```python
from build123d import *

# Parameters (mm, degrees)
EXTRUDE_1_DEPTH     = 6.5
SKETCH_2_R          = 8.75
EXTRUDE_2_DEPTH     = 3
SKETCH_3_R          = 10
EXTRUDE_3_DEPTH     = 12.5
CHAMFER_1_SIZE      = 1.5
SKETCH_6_R          = 5
CUT_EXTRUDE_1_DEPTH = 29.172880507
CHAMFER_2_SIZE      = 0.5


with BuildPart() as part:
    # 草图1 → 凸台-拉伸1 (new body)
    with BuildSketch(Plane(origin=(0, 0, 0), x_dir=(1, 0, 0), z_dir=(0, 1, 0))):
        Polygon((6.553289027, 11.549360859), (-6.725395388, 11.449995205), (-13.278684415, -0.099365654), (-6.553289027, -11.549360859), (6.725395388, -11.449995205), (13.278684415, 0.099365654), align=None)
    extrude(amount=EXTRUDE_1_DEPTH)

    # 草图2 → 凸台-拉伸2 (add)
    with BuildSketch(Plane(origin=(0, 6.5, 0), x_dir=(1, 0, 0), z_dir=(0, 1, 0))):
        with Locations(Location((0, 0, 0), (0, 0, 270))):
            Circle(SKETCH_2_R)
    extrude(amount=EXTRUDE_2_DEPTH)

    # 草图3 → 凸台-拉伸3 (add)
    with BuildSketch(Plane(origin=(0, 9.5, 0), x_dir=(1, 0, 0), z_dir=(0, 1, 0))):
        with Locations(Location((0, 0, 0), (0, 0, 270))):
            Circle(SKETCH_3_R)
    extrude(amount=EXTRUDE_3_DEPTH)

    # 倒角1
    chamfer_1_edges = [part.edges().sort_by_distance(p)[0] for p in [
        (0, 22, -10),
    ]]
    chamfer(chamfer_1_edges, length=CHAMFER_1_SIZE)

    # 草图5 → 切除-旋转3 (revolve, cut)
    with BuildSketch(Plane(origin=(0, 0, 0), x_dir=(0.49350563267132574, 0, -0.8697426001534446), z_dir=(0.8697426001534445, 0, 0.4935056326713257)), mode=Mode.PRIVATE) as cut_revolve_3_sk:
        Polygon((13.279056191, 1), (11.279056191, 0), (13.279056191, 0), align=None)
    revolve(cut_revolve_3_sk.sketch.rotate(Axis((0, -1000, 0), (0, 1, 0)), 180.000000003), axis=Axis((0, -1000, 0), (0, 1, 0)), mode=Mode.SUBTRACT)

    # 草图6 → 切除-拉伸1 (cut, through all)
    with BuildSketch(Plane(origin=(0, 22, 0), x_dir=(1, 0, 0), z_dir=(0, 1, 0))):
        with Locations(Location((0, 0, 0), (0, 0, 270))):
            Circle(SKETCH_6_R)
    extrude(amount=-CUT_EXTRUDE_1_DEPTH, mode=Mode.SUBTRACT)

    # 倒角2
    chamfer_2_edges = [part.edges().sort_by_distance(p)[0] for p in [
        (0, 0, -5),
        (0, 22, -5),
    ]]
    chamfer(chamfer_2_edges, length=CHAMFER_2_SIZE)


solid = part.part
```
Verification items for the finished model (mm, model axes). A direction names the side the tool comes from. Round coordinates to 2 decimals unless told otherwise and drop trailing zeros. Write each loop counter-clockwise with the first axis right and the second up, starting at its lowest first coordinate (ties: lowest second). Pieces come first, ordered by that corner, then holes.
1. Access from +Z, -Z, +X, -X, +Y, -Y to the whole of each face (thin tool, end or side, straight path). Record for faces 1 (the cylindrical face through (-9.76, 14.92, -2.17)), 2 (the cylindrical face through (-5.324, 7.979, -6.944)), 3 (the flat face through (-6, 22, 0)).
2. Section check B-B on x = 0. Enter the section's corners in (y, z).
3. Section check C-C on y = 10.5. Enter the section's corners in (x, z), plus the area to 3 significant figures.
4. Scan lines: L1, parallel to X at y = 14, z = 0; L2, parallel to X at y = 9.25, z = 0; L3, parallel to Y at x = -8.5, z = -4.5. Record each from-to range of solid material in increasing order.
5. Draft check along Z on faces 4 (the flat face through (-9.963, 3.261, 5.744)), 5 (the flat face through (-9, 9.5, 0)), 6 (the cylindrical face through (-4.88, 11.15, -1.08)). Enter one of: +Z half, -Z half, draft (parallel to the pull), parting line (faces both ways), or undercut.
6. Section check A-A on y = 5.5. Enter the section's corners in (x, z).
7. Gauge pin test, flat ends, axial feed: P1, Ø1.5, axis at y = 6, z = -6, coming from the +X side; P2, Ø10, axis at y = 6, z = -7, coming from the +X side; P3, Ø6, axis at x = 7, y = 15, coming from the +Z side. Record the tip position at first contact, or that the pin passes through.
Answer:
1. face 1: +Y
1. face 2: none
1. face 3: +Z, -Z, +X, -X, +Y
2. outline: (0, -11.28) - (0.11, -11.5) - (6.5, -11.5) - (6.5, -8.75) - (9.5, -8.75) - (9.5, -10) - (20.5, -10) - (22, -8.5) - (22, -5.5) - (21.5, -5) - (0.5, -5) - (0, -5.5) - close; (0, 5.5) - (0.5, 5) - (21.5, 5) - (22, 5.5) - (22, 8.5) - (20.5, 10) - (9.5, 10) - (9.5, 8.75) - (6.5, 8.75) - (6.5, 11.5) - (0.11, 11.5) - (0, 11.28) - close
3. outline: circle Ø20 at (0, 0); hole circle Ø10 at (0, 0)
3. area: 236 mm2
4. L1: x = -10 to -5, 5 to 10
4. L2: x = -8.75 to -5, 5 to 8.75
4. L3: y = 0 to 6.5, 9.5 to 20.88
5. face 4: +Z half
5. face 5: draft
5. face 6: undercut
6. outline: (-13.28, 0.1) - (-6.73, -11.45) - (6.55, -11.55) - (13.28, -0.1) - (6.73, 11.45) - (-6.55, 11.55) - close; hole circle Ø10 at (0, 0)
7. P1: stops at x = 10.25
7. P2: stops at x = 12.16
7. P3: stops at z = 9.17
